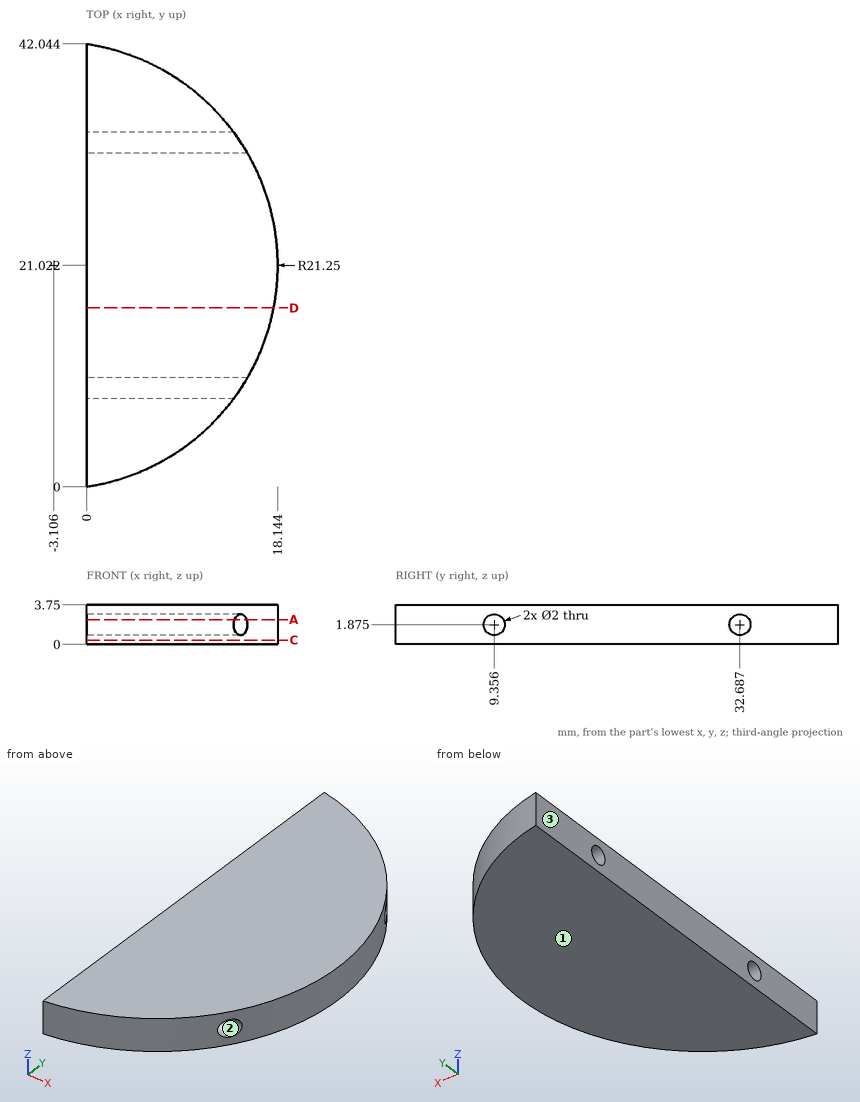
Part print with two shaded views. Sizes in mm from the minimum x, y, z corner. Coordinates: 2 decimals unless noted, no trailing zeros. Write each loop counter-clockwise with the first axis right and the second up, starting at its lowest first coordinate (ties: lowest second). Pieces come first, ordered by that corner, then holes.
(1) Cut at A-A on z = 2.35. State how many separate pieces and enclosed holes the cut face has, and give its area (3 significant figures).
(2) Cut at C-C on z = 0.4. List the corners of the cut face in (x, y).
(3) Drill centre lines: line 1 (X direction, y = 21.5, z = 2.8); line 2 (Y direction, x = 9.5, z = 1.7) (1 decimal); line 3 (Z direction, x = 5.5, y = 9). Where is each one in solid material? Low to high.
(4) Mould opens along Z. For the marked faces 1, 2 and 3 say: pulls with the +Z half, pulls with the -Z half, needs draft (parallel to the pull), parting line crosses it, or undercut.
(5) Pin check, flat tips, straight feed: pin 1 Ø1 at (y, z) = (14, 2) entering from +X; pin 2 Ø1.6 at (y, z) = (32.69, 1.88) entering from -X (3 decimals); pin 3 Ø1 at (y, z) = (22.5, 2) entering from +X. Stop position of each tip, or through.
(6) Cut at D-D on y = 17. List the corners of the cut face in (x, z).
Working result:
1. separate pieces: 3
1. enclosed holes: 0
1. area: 526 mm2
2. outline: (0, 0) arc R21.25 ccw to (0, 42.04) - close
3. line 1: x = 0 to 18.14
3. line 2: y = 3.9 to 8.4, 10.3 to 31.7, 33.7 to 38.1
3. line 3: z = 0 to 0.94, 2.81 to 3.75
4. face 1: pulls with the -Z half
4. face 2: undercut
4. face 3: needs draft
5. pin 1: stops at x = 17.12
5. pin 2: passes through
5. pin 3: stops at x = 18.12
6. outline: (0, 0) - (17.76, 0) - (17.76, 3.75) - (0, 3.75) - close
